Here's the drawing with two shaded views (mm, measured from the low corner). I have some questions. A direction names the side the tool comes from. Give positions to 0.01 mm unless a question says otherwise; leave off trailing zeros. Write each loop counter-clockwise with the first axis right and the second up, starting at its lowest first coordinate (ties: lowest second). Pieces come first, ordered by that corner, then holes. Notation, with made-up numbers: (76.25, 13.5) - (96.25, 13.5) arc R31 cw to (96.25, 46.5) - close; hole circle Ø11 at (72, 9). An arc over 180 degrees is marked (long way). Use one line per item in the form item = value. Start each with the question number.
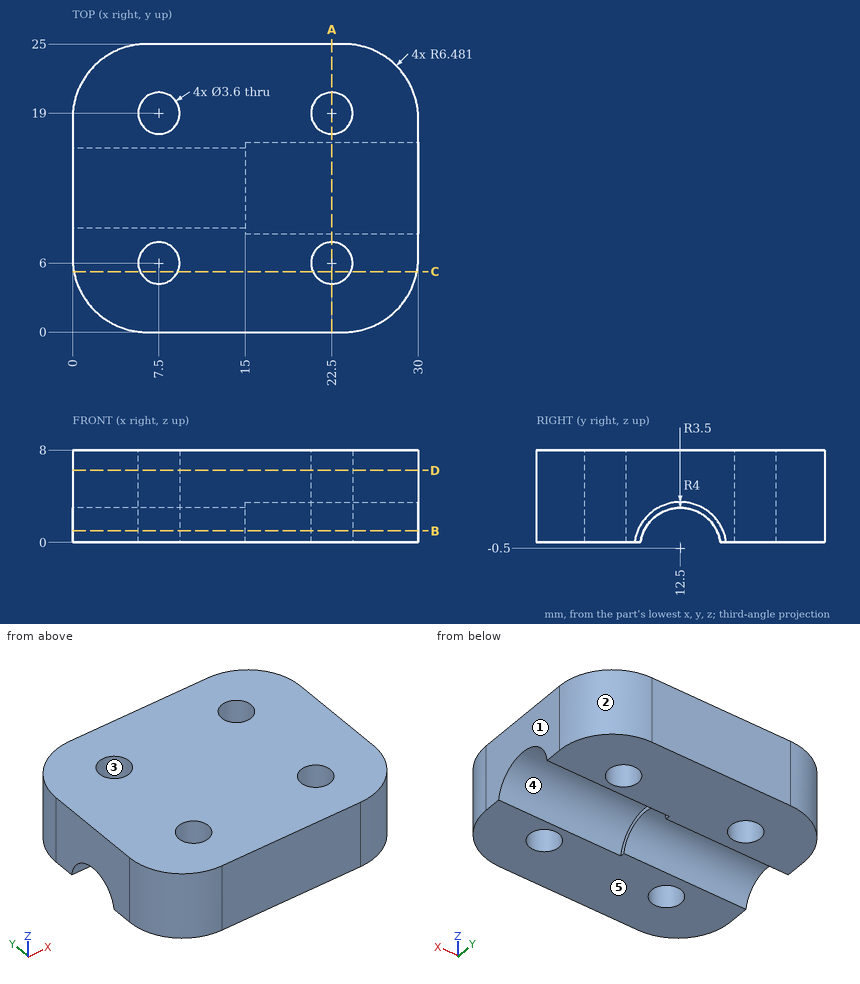
1. For the marked faces 4 and 5, which set-ups out of +Z, -Z, +X, -X, +Y, -Y let a thin tool reach every point of the face, with its end or its side?
2. I want a section at D-D, the plane z = 6.25. List the corners of the cut face in (x, y) for me, then the cut area to 3 significant figures.
3. I want a section at B-B, the plane z = 1. List the corners of the cut face in (x, y) for me, then the cut area to 3 significant figures.
4. Please list where these lines run through material, in increasing order: line 1 (Y direction, x = 7.5, z = 6); line 2 (Y direction, x = 21, z = 5) (1 decimal); line 3 (X direction, y = 4.5, z = 7) (1 decimal).
5. I want a section at C-C, the plane y = 5.25. List the corners of the cut face in (x, z) for me.
6. I want a section at A-A, the plane x = 22.5. List the corners of the cut face in (y, z) for me.
7. For P1, Ø4, axis at x = 7.5, y = 19, coming from the -Z side, with a flat end and sliding along its axis, tell me the tip position at first contact or that it passes through.
8. We'd pull the mould along Y, two halves only. Please class the marked faces 1, 2 and 3: pulls with the +Y half, pulls with the -Y half, needs draft (parallel to the pull), parting line crosses it, or undercut.
Result sheet:
q1.face_4 = -Z, +X
q1.face_5 = -Z, +X, -X, +Y, -Y
q2.outline = (0, 6.48) arc R6.48 ccw to (6.48, 0) - (23.52, 0) arc R6.48 ccw to (30, 6.48) - (30, 18.52) arc R6.48 ccw to (23.52, 25) - (6.48, 25) arc R6.48 ccw to (0, 18.52) - close; hole circle Ø3.6 at (7.5, 6); hole circle Ø3.6 at (7.5, 19); hole circle Ø3.6 at (22.5, 6); hole circle Ø3.6 at (22.5, 19)
q2.area = 673 mm2
q3.outline = (0, 6.48) arc R6.48 ccw to (6.48, 0) - (23.52, 0) arc R6.48 ccw to (30, 6.48) - (30, 8.79) - (15, 8.79) - (15, 9.34) - (0, 9.34) - close; (0, 15.66) - (15, 15.66) - (15, 16.21) - (30, 16.21) - (30, 18.52) arc R6.48 ccw to (23.52, 25) - (6.48, 25) arc R6.48 ccw to (0, 18.52) - close; hole circle Ø3.6 at (7.5, 6); hole circle Ø3.6 at (7.5, 19); hole circle Ø3.6 at (22.5, 6); hole circle Ø3.6 at (22.5, 19)
q3.area = 467 mm2
q4.line_1 = 0 to 4.2, 7.8 to 17.2, 20.8 to 25
q4.line_2 = 0 to 5, 7 to 18, 20 to 25
q4.line_3 = 0.3 to 6.5, 8.5 to 21.5, 23.5 to 29.7
q5.outline = (0.12, 0) - (5.86, 0) - (5.86, 8) - (0.12, 8) - close; (9.14, 0) - (20.86, 0) - (20.86, 8) - (9.14, 8) - close; (24.14, 0) - (29.88, 0) - (29.88, 8) - (24.14, 8) - close
q6.outline = (0, 0) - (4.2, 0) - (4.2, 8) - (0, 8) - close; (7.8, 0) - (8.53, 0) arc R4 cw to (16.47, 0) - (17.2, 0) - (17.2, 8) - (7.8, 8) - close; (20.8, 0) - (25, 0) - (25, 8) - (20.8, 8) - close
q7.P1 = 0
q8.face_1 = needs draft
q8.face_2 = pulls with the +Y half
q8.face_3 = undercut
